Verification items for this drawing (mm, ordinates from the low corner). Give positions to 0.01 mm unless a question says otherwise; leave off trailing zeros. Order: outer loops, then holes, each group sorted by start corner. A loop starts at its lowest first (then second) coordinate and runs counter-clockwise, first axis right, second up. Notation, with made-up numbers: (63.25, 77) -> (105.25, 77) arc R20 cw to (105.25, 92) -> close; hole circle Ø4 at (-11.75, 88.25). An arc over 180 degrees is marked (long way). One line per question, with ' | ' between items.
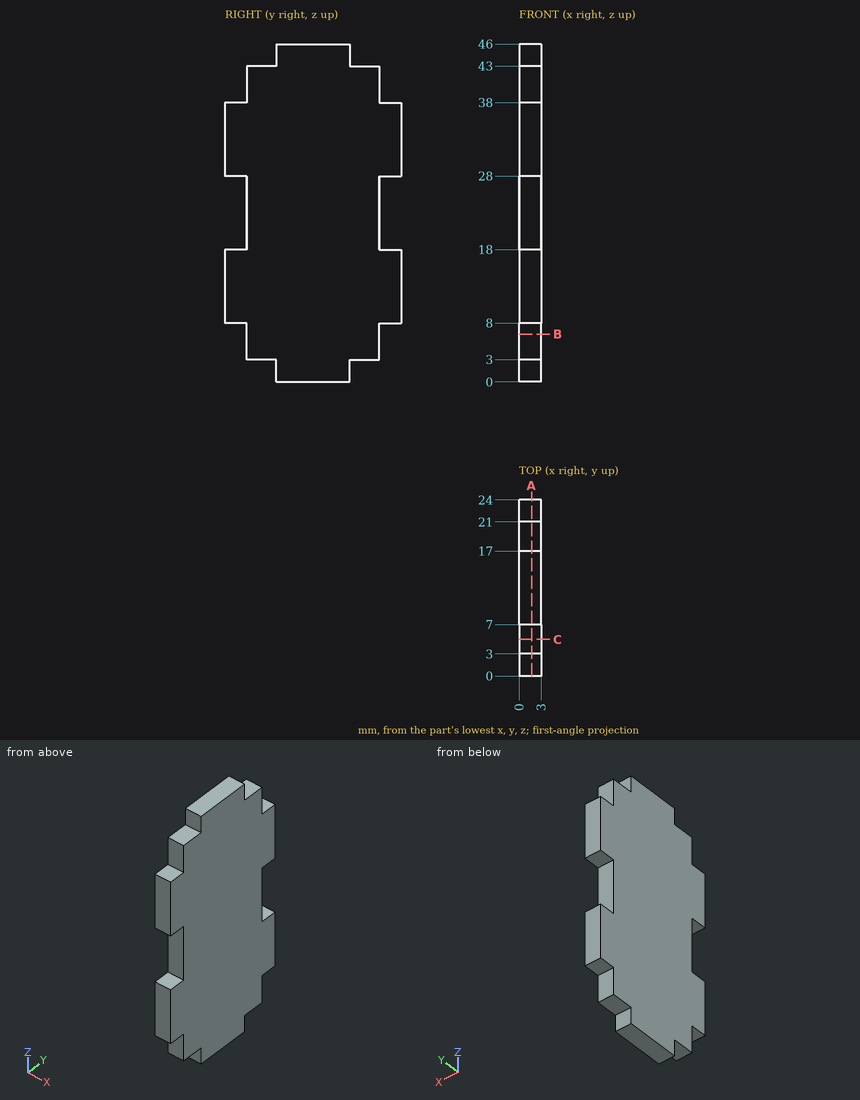
Q1. Section check B-B (z = 6.5). Enter the section's corners in (x, y), and give its area (3 significant figures).
Result sheet:
outline: (0, 3) -> (3, 3) -> (3, 21) -> (0, 21) -> close | area: 54.0 mm2
Q2. Thickness scan on line 1 (Y direction, x = 2.2, z = 7.5); line 2 (Z direction, x = 0.5, y = 6); line 3 (Y direction, x = 1.1, z = 2.5). Record the ranges inside material, lowest first.
Result sheet:
line 1: y = 3 to 21 | line 2: z = 3 to 43 | line 3: y = 7 to 17
Q3. Section check C-C (y = 5). Enter the section's corners in (x, z).
Result sheet:
outline: (0, 3) -> (3, 3) -> (3, 43) -> (0, 43) -> close
Q4. Section check A-A (x = 1.7). Enter the section's corners in (y, z).
Result sheet:
outline: (0, 8) -> (3, 8) -> (3, 3) -> (7, 3) -> (7, 0) -> (17, 0) -> (17, 3) -> (21, 3) -> (21, 8) -> (24, 8) -> (24, 18) -> (21, 18) -> (21, 28) -> (24, 28) -> (24, 38) -> (21, 38) -> (21, 43) -> (17, 43) -> (17, 46) -> (7, 46) -> (7, 43) -> (3, 43) -> (3, 38) -> (0, 38) -> (0, 28) -> (3, 28) -> (3, 18) -> (0, 18) -> close
Q5. Depth check by flat-ended pin: pin 1 Ø1.5 at (x, y) = (1, 22.5) entering from +Z; pin 2 Ø1.5 at (x, z) = (1.5, 41) entering from +Y; pin 3 Ø0.9 at (x, z) = (1, 1.5) entering from -Y. Enter the tip coordinate at first touch or a pass-through.
Result sheet:
pin 1: stops at z = 38 | pin 2: stops at y = 21 | pin 3: stops at y = 7
